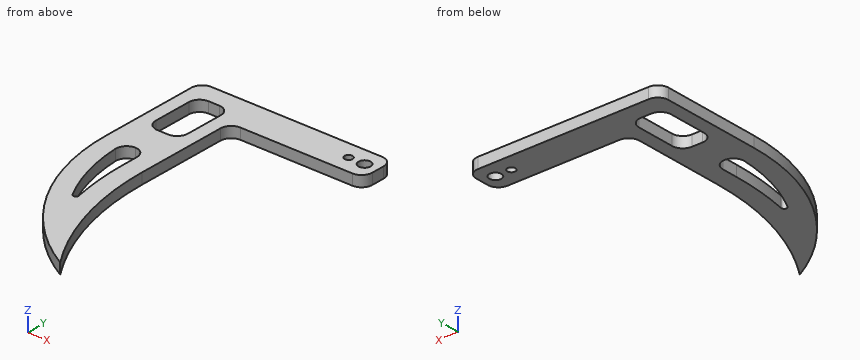
```python
from build123d import *

# Parameters (mm, degrees)
ESQUISSE1_W             = 12
ESQUISSE1_H             = 22.5
BOSS_EXTRU_1_DEPTH      = 4
ENL_V_MAT_EXTRU_1_DEPTH = 94.445721179
SKETCH1_W               = 50
SKETCH1_H               = 13
BOSS_EXTRUDE1_DEPTH     = 4
SKETCH2_R               = 2.25
SKETCH2_R_2             = 1.5
CUT_EXTRUDE1_DEPTH      = 4
FILLET1_R               = 4
FILLET2_R               = 1


with BuildPart() as part:
    # Esquisse1 → Boss.-Extru.1 (new body)
    with BuildSketch(Plane.XY):
        with BuildLine():
            Line((-11, -18.25), (-11, 18.25))
            Line((-11, 18.25), (11, 18.25))
            Line((11, 18.25), (11, -18.25))
            Line((11, -18.25), (11, -33.25))
            ThreePointArc((11, -33.25), (15.349591107, -62.421891926), (28.019985571, -89.056067818))
            ThreePointArc((28.019985571, -89.056067818), (-0.511631053, -61.502443829), (-11, -23.25))
            Line((-11, -23.25), (-11, -18.25))
        make_face()
        Rectangle(ESQUISSE1_W, ESQUISSE1_H, mode=Mode.SUBTRACT)
    extrude(amount=BOSS_EXTRU_1_DEPTH)

    # Esquisse2 → Enlèv. mat.-Extru.1 (cut, through all)
    with BuildSketch(Plane.XY.offset(4)):
        with BuildLine():
            Line((-4, -23.25), (4, -23.25))
            Line((4, -23.25), (4, -33.25))
            ThreePointArc((4, -33.25), (4.956601419, -47.525770288), (7.809301258, -61.546284087))
            ThreePointArc((7.809301258, -61.546284087), (-0.980641404, -43.287870216), (-4, -23.25))
        make_face()
    extrude(amount=-ENL_V_MAT_EXTRU_1_DEPTH, mode=Mode.SUBTRACT)

    # Sketch1 → Boss-Extrude1 (add)
    with BuildSketch(Plane.XY.offset(4)):
        with Locations((36, 11.75)):
            Rectangle(SKETCH1_W, SKETCH1_H)
    extrude(amount=-BOSS_EXTRUDE1_DEPTH)

    # Sketch2 → Cut-Extrude1 (cut)
    with BuildSketch(Plane.XY.offset(4)):
        with Locations((56, 11.75)):
            Circle(SKETCH2_R)
        with Locations((50, 11.75)):
            Circle(SKETCH2_R_2)
    extrude(amount=-CUT_EXTRUDE1_DEPTH, mode=Mode.SUBTRACT)

    # Fillet1
    # the kernel refuses this fillet: 4 mm, written as the material it adds along each edge
    with BuildSketch(Plane(origin=(11, 5.25, 4), x_dir=(0, -1, 0), z_dir=(0, 0, -1)), Plane(origin=(4, -23.25, 4), x_dir=(-1, 0, 0), z_dir=(0, 0, -1)), Plane(origin=(6, -11.25, 0), x_dir=(-1, 0, 0), z_dir=(0, 0, 1)), Plane(origin=(6, 11.25, 0), x_dir=(0, -1, 0), z_dir=(0, 0, 1))) as fillet1_piece_1:
        with BuildLine():
            CenterArc((FILLET1_R, -FILLET1_R), FILLET1_R, 90, 90)
            Line((0, -FILLET1_R), (0, 0))
            Line((0, 0), (FILLET1_R, 0))
        make_face()
    extrude(amount=4)
    with BuildSketch(Plane(origin=(-4, -23.25, 4), x_dir=(1, 0, 0), z_dir=(0, 0, -1))) as fillet1_piece_2:
        with BuildLine():
            CenterArc((4.125122309, 4), FILLET1_R, 176.416678302, 93.583321698)
            ThreePointArc((0.132942454, 4.25), (0.033243739, 2.126039375), (0, 0))
            Line((0, 0), (4.125122309, 0))
        make_face()
    extrude(amount=4)
    with BuildSketch(Plane(origin=(-6, -11.25, 0), x_dir=(1, 0, 0), z_dir=(0, 0, 1)), Plane(origin=(-6, 11.25, 0), x_dir=(0, -1, 0), z_dir=(0, 0, 1))) as fillet1_piece_3:
        with BuildLine():
            CenterArc((FILLET1_R, FILLET1_R), FILLET1_R, 180, 90)
            Line((0, FILLET1_R), (0, 0))
            Line((0, 0), (FILLET1_R, 0))
        make_face()
    extrude(amount=4)
    # the kernel refuses this fillet: 4 mm, written as the material it takes off along each edge
    with BuildSketch(Plane(origin=(-11, 18.25, -10), x_dir=(0, -1, 0), z_dir=(0, 0, 1))) as fillet1_2_piece_1:
        with BuildLine():
            CenterArc((FILLET1_R, FILLET1_R), FILLET1_R, 180, 90)
            Line((0, FILLET1_R), (0, 0))
            Line((0, 0), (FILLET1_R, 0))
        make_face()
    extrude(amount=24, mode=Mode.SUBTRACT)
    with BuildSketch(Plane(origin=(61, 5.25, 14), x_dir=(0, 1, 0), z_dir=(0, 0, -1)), Plane(origin=(61, 18.25, 14), x_dir=(-1, 0, 0), z_dir=(0, 0, -1))) as fillet1_2_piece_2:
        with BuildLine():
            CenterArc((FILLET1_R, -FILLET1_R), FILLET1_R, 90, 90)
            Line((0, -FILLET1_R), (0, 0))
            Line((0, 0), (FILLET1_R, 0))
        make_face()
    extrude(amount=24, mode=Mode.SUBTRACT)

    # Fillet2
    fillet2_edges = [part.edges().sort_by_distance(p)[0] for p in [
        (7.809301258, -61.546284087, 2),
    ]]
    fillet(fillet2_edges, radius=FILLET2_R)


solid = part.part
```
CAD build for the part. Positions are in the model's coordinates, mm. Round coordinates to 2 decimals unless told otherwise and drop trailing zeros. Order: outer loops, then holes, each group sorted by start corner. A loop starts at its lowest first (then second) coordinate and runs counter-clockwise, first axis right, second up.
Q1. Slice it at C-C (z = 1.95). State how many separate pieces and enclosed holes the cut face has, and give its area (3 significant figures).
Q2. Drop flat-ended pins along their axis: pin 1 (1 mm diameter, centred on y = -5.5, z = 2.5, fed in from +X); pin 2 (2 mm diameter, centred on x = 53, z = 3, fed in from -Y); pin 3 (1.5 mm diameter, centred on y = -43, z = 2.5, fed in from +X). Give the stop position or say it passes through.
Q3. Wall check: L1, parallel to Y at x = 56, z = 1.2; L2, parallel to X at y = 0, z = 3.8; L3, parallel to Y at x = 3, z = 1.35. Give the ranges that are in metal, low to high.
Q4. Slice it at B-B (y = -53). Write the cut outline in (x, z).
Q5. Slice it at D-D (x = 34). Write the cut outline in (y, z), and give its area (3 significant figures).
Q6. Slice it at A-A (x = 50). Write the cut outline in (y, z).
Results below:
1. separate pieces: 1
1. enclosed holes: 4
1. area: 2,100 mm2
2. pin 1: stops at x = 11
2. pin 2: stops at y = 5.25
2. pin 3: stops at x = 11.55
3. L1: y = 5.25 to 9.5, 14 to 18.25
3. L2: x = -11 to -6, 6 to 11
3. L3: y = -66.88 to -53.3, -24.6 to -11.12, 11.12 to 18.25
4. outline: (-4.85, 0) - (2.85, 0) - (2.85, 4) - (-4.85, 4) - close; (5.84, 0) - (12.97, 0) - (12.97, 4) - (5.84, 4) - close
5. outline: (5.25, 0) - (18.25, 0) - (18.25, 4) - (5.25, 4) - close
5. area: 52.0 mm2
6. outline: (5.25, 0) - (10.25, 0) - (10.25, 4) - (5.25, 4) - close; (13.25, 0) - (18.25, 0) - (18.25, 4) - (13.25, 4) - close
